from build123d import *

# Parameters (mm, degrees)
SKETCH1_W                       = 45
SKETCH1_H                       = 27
BOSS_EXTRUDE1_DEPTH             = 3
CUT_EXTRUDE1_REACH              = 28.41
SKETCH2_R                       = 1.75
SKETCH3_R                       = 3
CUT_EXTRUDE2_DEPTH              = 2
BOSS_EXTRUDE2_DEPTH             = 6
CUT_EXTRUDE6_REACH              = 37.992
CUT_EXTRUDE6_START              = -3
SKETCH12_R                      = 8.25
SKETCH15_R                      = 2.5
CUT_EXTRUDE7_DEPTH              = 6
SKETCH16_R                      = 1.15
SKETCH16_R_2                    = 12
BOSS_EXTRUDE5_DEPTH             = 2.5
CUT_EXTRUDE8_START              = -3.75
SKETCH17_W                      = 5.5
SKETCH17_H                      = 3
CUT_EXTRUDE8_DEPTH              = 82.37731478
BOSS_EXTRUDE6_START             = -9
SKETCH18_R                      = 1.75
BOSS_EXTRUDE6_DEPTH             = 5
SKETCH21_W                      = 11.5
SKETCH21_H                      = 33.5
SKETCH21_R                      = 1.75
BOSS_EXTRUDE7_DEPTH             = 5.5
CUT_EXTRUDE9_DEPTH              = 2
CHAMFER1_SIZE                   = 3
CHAMFER1_SIZE2                  = 5.196152423
FILLET1_R                       = 5
CUT_EXTRUDE10_REACH             = 74.347
SKETCH20_W                      = 4
SKETCH20_H                      = 8
CUT_EXTRUDE10_DIRECTION_2_DEPTH = 73.346820939
CHAMFER2_SIZE2                  = 3
CHAMFER2_SIZE                   = 20
CHAMFER3_SIZE2                  = 20
CHAMFER3_SIZE                   = 3


# Some blends are built 0.0001 mm under size
with BuildPart() as part:
    # Sketch1 → Boss-Extrude1 (new body)
    with BuildSketch(Plane(origin=(0, 0, 0), x_dir=(1, 0, 0), z_dir=(0, 1, 0))):
        Rectangle(SKETCH1_W, SKETCH1_H)
    extrude(amount=BOSS_EXTRUDE1_DEPTH)

    # Sketch2 → Cut-Extrude1 (cut, up to next)
    with BuildSketch(Plane(origin=(0, 3, 0), x_dir=(1, 0, 0), z_dir=(0, 1, 0)), mode=Mode.PRIVATE) as cut_extrude1_sk1:
        with Locations(Location((-10, 10, 0), (0, 0, 270))):
            Circle(SKETCH2_R)
    cut_extrude1_tool1 = extrude(cut_extrude1_sk1.sketch, amount=-CUT_EXTRUDE1_REACH, mode=Mode.PRIVATE) & part.part
    # Sketch2 → Cut-Extrude1 (cut, up to next)
    with BuildSketch(Plane(origin=(0, 3, 0), x_dir=(1, 0, 0), z_dir=(0, 1, 0)), mode=Mode.PRIVATE) as cut_extrude1_sk2:
        with Locations(Location((10, 10, 0), (0, 0, 270))):
            Circle(SKETCH2_R)
    cut_extrude1_tool2 = extrude(cut_extrude1_sk2.sketch, amount=-CUT_EXTRUDE1_REACH, mode=Mode.PRIVATE) & part.part
    # Sketch2 → Cut-Extrude1 (cut, up to next)
    with BuildSketch(Plane(origin=(0, 3, 0), x_dir=(1, 0, 0), z_dir=(0, 1, 0)), mode=Mode.PRIVATE) as cut_extrude1_sk3:
        with Locations(Location((10, -10, 0), (0, 0, 270))):
            Circle(SKETCH2_R)
    cut_extrude1_tool3 = extrude(cut_extrude1_sk3.sketch, amount=-CUT_EXTRUDE1_REACH, mode=Mode.PRIVATE) & part.part
    # Sketch2 → Cut-Extrude1 (cut, up to next)
    with BuildSketch(Plane(origin=(0, 3, 0), x_dir=(1, 0, 0), z_dir=(0, 1, 0)), mode=Mode.PRIVATE) as cut_extrude1_sk4:
        with Locations(Location((-10, -10, 0), (0, 0, 270))):
            Circle(SKETCH2_R)
    cut_extrude1_tool4 = extrude(cut_extrude1_sk4.sketch, amount=-CUT_EXTRUDE1_REACH, mode=Mode.PRIVATE) & part.part
    add(cut_extrude1_tool1.solids().sort_by_distance((-10, 3, -10))[0], mode=Mode.SUBTRACT)
    add(cut_extrude1_tool2.solids().sort_by_distance((10, 3, -10))[0], mode=Mode.SUBTRACT)
    add(cut_extrude1_tool3.solids().sort_by_distance((10, 3, 10))[0], mode=Mode.SUBTRACT)
    add(cut_extrude1_tool4.solids().sort_by_distance((-10, 3, 10))[0], mode=Mode.SUBTRACT)

    # Sketch3 → Cut-Extrude2 (cut)
    with BuildSketch(Plane(origin=(0, 3, 0), x_dir=(1, 0, 0), z_dir=(0, 1, 0))):
        with Locations(Location((-10, 10, 0), (0, 0, 270))):
            Circle(SKETCH3_R)
        with Locations(Location((10, 10, 0), (0, 0, 90))):
            Circle(SKETCH3_R)
        with Locations(Location((10, -10, 0), (0, 0, 270))):
            Circle(SKETCH3_R)
        with Locations(Location((-10, -10, 0), (0, 0, 90))):
            Circle(SKETCH3_R)
    extrude(amount=-CUT_EXTRUDE2_DEPTH, mode=Mode.SUBTRACT)

    # Sketch5 → Boss-Extrude2 (add, symmetric)
    with BuildSketch(Plane.XY):
        with BuildLine():
            Line((16.25, 3), (-16.25, 3))
            Line((-16.25, 3), (-16.25, 20))
            Line((-16.25, 20), (-6.25, 20))
            ThreePointArc((-6.25, 20), (0, 13.75), (6.25, 20))
            Line((6.25, 20), (16.25, 20))
            Line((16.25, 20), (16.25, 3))
        make_face()
    extrude(amount=BOSS_EXTRUDE2_DEPTH, both=True)

    # Sketch12 → Cut-Extrude6 (cut, up to next)
    with BuildSketch(Plane.XY.offset(CUT_EXTRUDE6_START), mode=Mode.PRIVATE) as cut_extrude6_sk1:
        with Locations((0, 20)):
            Circle(SKETCH12_R)
    cut_extrude6_tool1 = extrude(cut_extrude6_sk1.sketch, amount=-CUT_EXTRUDE6_REACH, mode=Mode.PRIVATE) & part.part
    cut_extrude6 = cut_extrude6_tool1.solids().sort_by_distance((0, 20, -3))[0]
    add(cut_extrude6, mode=Mode.SUBTRACT)

    # Mirror1: Cut-Extrude6 across plane
    add(cut_extrude6.mirror(Plane.XY), mode=Mode.SUBTRACT)

    # Sketch15 → Cut-Extrude7 (cut)
    with BuildSketch(Plane(origin=(0, 20, 0), x_dir=(1, 0, 0), z_dir=(0, 1, 0))):
        with Locations(Location((-11.25, 0, 0), (0, 0, 180))):
            Circle(SKETCH15_R)
        with Locations((11.25, 0)):
            Circle(SKETCH15_R)
    extrude(amount=-CUT_EXTRUDE7_DEPTH, mode=Mode.SUBTRACT)

    # Sketch16 → Boss-Extrude5 (add)
    with BuildSketch(Plane.ZY.offset(16.25)):
        Polygon((9, 3), (9, 0), (49, 0), (49, 40), (9, 40), (6, 40), (6, 20), (-6, 20), (-6, 3), align=None)
        with Locations((47, 2)):
            Circle(SKETCH16_R, mode=Mode.SUBTRACT)
        with Locations(Location((47, 38, 0), (0, 0, 180))):
            Circle(SKETCH16_R, mode=Mode.SUBTRACT)
        with Locations(Location((11, 38, 0), (0, 0, 180))):
            Circle(SKETCH16_R, mode=Mode.SUBTRACT)
        with Locations((29, 20)):
            Circle(SKETCH16_R_2, mode=Mode.SUBTRACT)
    boss_extrude5 = extrude(amount=BOSS_EXTRUDE5_DEPTH)

    # Sketch17 → Cut-Extrude8 (cut)
    with BuildSketch(Plane.ZY.offset(22.5).offset(CUT_EXTRUDE8_START)):
        with Locations((10.75, 1.5)):
            Rectangle(SKETCH17_W, SKETCH17_H)
    cut_extrude8 = extrude(amount=CUT_EXTRUDE8_DEPTH, mode=Mode.SUBTRACT)

    # Mirror2: Boss-Extrude5, Cut-Extrude8 across plane
    add(boss_extrude5.mirror(Plane(origin=(0, 0, 0), x_dir=(0, 0, 1), z_dir=(1, 0, 0))))
    add(cut_extrude8.mirror(Plane(origin=(0, 0, 0), x_dir=(0, 0, 1), z_dir=(1, 0, 0))), mode=Mode.SUBTRACT)

    # Sketch18 → Boss-Extrude6 (add)
    with BuildSketch(Plane(origin=(0, 0, -6), x_dir=(-1, 0, 0), z_dir=(0, 0, -1)).offset(BOSS_EXTRUDE6_START)):
        Polygon((-42.25, 33.5), (-30.75, 33.5), (-30.75, 6.5), (-18.75, 6.5), (-18.75, 0), (-42.25, 0), (-42.25, 6.5), align=None)
        with Locations((-36.5, 29)):
            Circle(SKETCH18_R, mode=Mode.SUBTRACT)
        with Locations(Location((-36.5, 11, 0), (0, 0, 180))):
            Circle(SKETCH18_R, mode=Mode.SUBTRACT)
    extrude(amount=-BOSS_EXTRUDE6_DEPTH)

    # Sketch21 → Boss-Extrude7 (add)
    with BuildSketch(Plane.XY.offset(8)):
        with Locations((36.5, 16.75)):
            Rectangle(SKETCH21_W, SKETCH21_H)
        with Locations(Location((36.5, 29, 0), (0, 0, 180))):
            Circle(SKETCH21_R, mode=Mode.SUBTRACT)
        with Locations((36.5, 11)):
            Circle(SKETCH21_R, mode=Mode.SUBTRACT)
    extrude(amount=BOSS_EXTRUDE7_DEPTH)

    # Sketch19 → Cut-Extrude9 (cut)
    with BuildSketch(Plane(origin=(0, 0, 3), x_dir=(-1, 0, 0), z_dir=(0, 0, -1))):
        Polygon((-39.848631561, 11), (-38.174315781, 8.1), (-34.825684219, 8.1), (-33.151368439, 11), (-34.825684219, 13.9), (-38.174315781, 13.9), align=None)
        Polygon((-39.848631561, 29), (-38.174315781, 26.1), (-34.825684219, 26.1), (-33.151368439, 29), (-34.825684219, 31.9), (-38.174315781, 31.9), align=None)
    extrude(amount=-CUT_EXTRUDE9_DEPTH, mode=Mode.SUBTRACT)

    # Chamfer1
    chamfer1_edges = [part.edges().sort_by_distance(p)[0] for p in [
        (42.25, 33.5, 8.25),
        (30.75, 33.5, 8.25),
    ]]
    chamfer1_side = [part.faces().sort_by_distance(p)[0] for p in [
        (36.5, 33.5, 8.25),
    ]]
    chamfer(chamfer1_edges, length=CHAMFER1_SIZE, length2=CHAMFER1_SIZE2, reference=chamfer1_side[0])

    # Fillet1
    # the kernel refuses this fillet: 5 mm, written as the material it takes off along each edge
    with BuildSketch(Plane(origin=(42.25, 0, -9.5), x_dir=(-1, 0, 0), z_dir=(0, 0, 1))) as fillet1_piece_1:
        with BuildLine():
            CenterArc((FILLET1_R, -FILLET1_R), FILLET1_R, 90, 90)
            Line((0, -FILLET1_R), (0, 0))
            Line((0, 0), (FILLET1_R, 0))
        make_face()
    extrude(amount=35.5, mode=Mode.SUBTRACT)
    with BuildSketch(Plane(origin=(42.25, 28.303847577, -0.349364905), x_dir=(-0.4999999999999988, 0.8660254037844394, 0), z_dir=(0, 0, 1))) as fillet1_piece_2:
        with BuildLine():
            CenterArc((FILLET1_R * 0.267949192431, FILLET1_R), FILLET1_R, 240, 30)
            Line((-FILLET1_R * 0.232050807569, FILLET1_R * 0.133974596216), (0, 0))
            Line((0, 0), (FILLET1_R * 0.267949192431, 0))
        make_face()
    extrude(amount=17.198729811, mode=Mode.SUBTRACT)
    with BuildSketch(Plane(origin=(30.75, 28.303847577, 16.849364905), x_dir=(0, -1, 0), z_dir=(0, 0, -1))) as fillet1_piece_3:
        with BuildLine():
            CenterArc((FILLET1_R * 0.267949192431, -FILLET1_R), FILLET1_R, 90, 30)
            Line((-FILLET1_R * 0.232050807569, -FILLET1_R * 0.133974596216), (0, 0))
            Line((0, 0), (FILLET1_R * 0.267949192431, 0))
        make_face()
    extrude(amount=17.198729811, mode=Mode.SUBTRACT)
    with BuildSketch(Plane(origin=(39.25, 33.5, -4.216878365), x_dir=(-1, 0, 0), z_dir=(0, 0, 1))) as fillet1_piece_4:
        with BuildLine():
            CenterArc((FILLET1_R * 0.57735026919, FILLET1_R), FILLET1_R, 210, 60)
            Line((-FILLET1_R * 0.288675134595, FILLET1_R * 0.5), (0, 0))
            Line((0, 0), (FILLET1_R * 0.57735026919, 0))
        make_face()
    extrude(amount=24.93375673, mode=Mode.SUBTRACT)
    with BuildSketch(Plane(origin=(33.75, 33.5, 20.716878365), x_dir=(-0.4999999999999974, -0.86602540378444, 0), z_dir=(0, 0, -1))) as fillet1_piece_5:
        with BuildLine():
            CenterArc((FILLET1_R * 0.57735026919, -FILLET1_R), FILLET1_R, 90, 60)
            Line((-FILLET1_R * 0.288675134595, -FILLET1_R * 0.5), (0, 0))
            Line((0, 0), (FILLET1_R * 0.57735026919, 0))
        make_face()
    extrude(amount=24.93375673, mode=Mode.SUBTRACT)

    # Sketch20 → Cut-Extrude10 (cut, up to next)
    with BuildSketch(Plane.XY.offset(6), mode=Mode.PRIVATE) as cut_extrude10_sk1:
        with Locations((-14.25, 7)):
            Rectangle(SKETCH20_W, SKETCH20_H)
    cut_extrude10_tool1 = extrude(cut_extrude10_sk1.sketch, amount=-CUT_EXTRUDE10_REACH, mode=Mode.PRIVATE) & part.part
    # Sketch20 → Cut-Extrude10 (cut, up to next)
    with BuildSketch(Plane.XY.offset(6), mode=Mode.PRIVATE) as cut_extrude10_sk2:
        with Locations((14.25, 7)):
            Rectangle(SKETCH20_W, SKETCH20_H)
    cut_extrude10_tool2 = extrude(cut_extrude10_sk2.sketch, amount=-CUT_EXTRUDE10_REACH, mode=Mode.PRIVATE) & part.part
    add(cut_extrude10_tool1.solids().sort_by_distance((-14.25, 7, 6))[0], mode=Mode.SUBTRACT)
    add(cut_extrude10_tool2.solids().sort_by_distance((14.25, 7, 6))[0], mode=Mode.SUBTRACT)

    # Sketch20 → Cut-Extrude10 direction 2 (cut)
    with BuildSketch(Plane.XY.offset(6)):
        with Locations((-14.25, 7)):
            Rectangle(SKETCH20_W, SKETCH20_H)
        with Locations((14.25, 7)):
            Rectangle(SKETCH20_W, SKETCH20_H)
    extrude(amount=CUT_EXTRUDE10_DIRECTION_2_DEPTH, mode=Mode.SUBTRACT)

    # Chamfer2
    chamfer2_edges = [part.edges().sort_by_distance(p)[0] for p in [
        (-17.5, 40, 6),
    ]]
    chamfer2_side = [part.faces().sort_by_distance(p)[0] for p in [
        (-17.5, 39.94, 6),
    ]]
    chamfer(chamfer2_edges, length=CHAMFER2_SIZE - 0.0001, length2=CHAMFER2_SIZE2 - 0.0001, reference=chamfer2_side[0])  # a hair under: the kernel refuses the full size

    # Chamfer3
    chamfer3_edges = [part.edges().sort_by_distance(p)[0] for p in [
        (17.5, 40, 6),
    ]]
    chamfer3_side = [part.faces().sort_by_distance(p)[0] for p in [
        (17.5, 40, 6.06),
    ]]
    chamfer(chamfer3_edges, length=CHAMFER3_SIZE - 0.0001, length2=CHAMFER3_SIZE2 - 0.0001, reference=chamfer3_side[0])  # a hair under: the kernel refuses the full size


solid = part.part
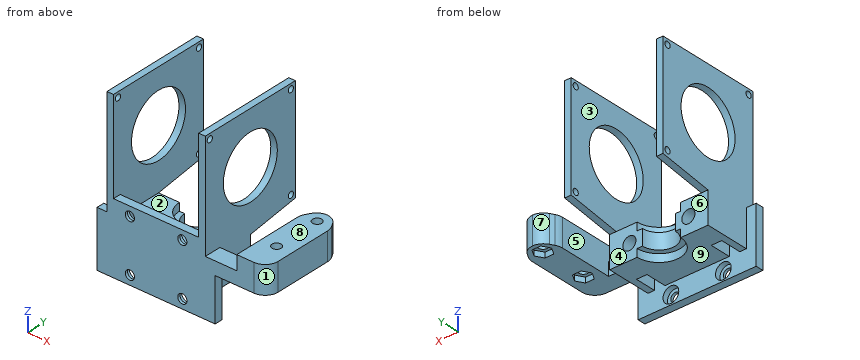
The model under review builds one solid part; all positions refer to its coordinate system, in mm. Face numbers are marked on the shaded views. A direction names the side the tool comes from. Coordinates: 2 decimals unless noted, no trailing zeros. Write each loop counter-clockwise with the first axis right and the second up, starting at its lowest first coordinate (ties: lowest second). Pieces come first, ordered by that corner, then holes. Notation, with made-up numbers: M -25.5,13.5 L 24.5,13.5 A21 ccw 24.5,49.5 Z; hole C 76.5,40.5 d7. An arc over 180 degrees is marked long. Put each result on its own line as item: value.
1) Add section B-B on z = 47. Give the boundary of the cut face in (x, y), then the cut area to 3 significant figures.
Computed:
outline: M -18.75,0 L -16.25,0 L -16.25,0.85 L -18.75,0.85 Z; M -18.75,3.15 L -16.25,3.15 L -16.25,36.85 L -18.75,36.85 Z; M -18.75,39.15 L -16.25,39.15 L -16.25,40 L -18.75,40 Z; M 16.25,0 L 18.75,0 L 18.75,0.85 L 16.25,0.85 Z; M 16.25,3.15 L 18.75,3.15 L 18.75,36.85 L 16.25,36.85 Z; M 16.25,39.15 L 18.75,39.15 L 18.75,40 L 16.25,40 Z
area: 177 mm2
2) Add section A-A on x = 10. Give the boundary of the cut face in (y, z), then the cut area to 3 significant figures.
Computed:
outline: M 0,-13.5 L 3,-13.5 L 3,-13 L 1,-13 L 1,-11.75 L 0,-11.75 Z; M 0,-8.25 L 1,-8.25 L 1,-7 L 3,-7 L 3,-6 L 20,-6 L 20,-2.17 L 14,-2.17 L 14,2.17 L 20,2.17 L 20,6 L 3,6 L 3,7 L 1,7 L 1,8.25 L 0,8.25 Z; M 0,11.75 L 1,11.75 L 1,13 L 3,13 L 3,13.5 L 0,13.5 Z
area: 228 mm2
3) For the marked faces 5, 6, 7, 8 and 9, list the 3-axis set-ups (+Z, -Z, +X, -X, +Y, -Y) from which the entire face can be reached by the end or side of a thin tool; tool diameter is ignored.
Computed:
face 5: +Z, +Y
face 6: -Z, -X, +Y
face 7: +Z, -Z, +Y
face 8: +Z, +X, +Y, -Y
face 9: -Z, +X, -X, +Y
4) Add section C-C on x = 0. Give the boundary of the cut face in (y, z), then the cut area to 3 significant figures.
Computed:
outline: M 0,-13.5 L 3,-13.5 L 3,-6 L 11.75,-6 L 11.75,-3 L 13.75,-3 L 13.75,3 L 11.75,3 L 11.75,6 L 3,6 L 3,13.5 L 0,13.5 Z
area: 198 mm2
5) Draft analysis for pull direction X (two halves, no side actions). For the marked faces 1, 2, 3 and 4, state which applies: released by +X, released by -X, zero draft, split by the parting line, or undercut.
Computed:
face 1: released by +X
face 2: undercut
face 3: undercut
face 4: zero draft
6) Wall thickness on probe 1 along X at (y, z) = (25, 13); probe 2 along X at (y, z) = (1.6, -10); probe 3 along Z at (x, y) = (10, 2): over which ranges is each line inside the solid? List them lowest first. Write a range as [from, to].
Computed:
probe 1: x = [-18.75, -16.25], [16.25, 18.75], [30.75, 42.25]
probe 2: x = [-22.5, -13], [-7, 7], [13, 22.5]
probe 3: z = [-13.5, -13], [-7, 7], [13, 13.5]
7) Add section D-D on y = 38. Give the boundary of the cut face in (x, z).
Computed:
outline: M -18.75,8.7 L -16.25,8.7 L -16.25,9.85 L -18.75,9.85 Z; M -18.75,12.15 L -16.25,12.15 L -16.25,45.85 L -18.75,45.85 Z; M -18.75,48.15 L -16.25,48.15 L -16.25,49 L -18.75,49 Z; M 16.25,8.7 L 18.75,8.7 L 18.75,9.85 L 16.25,9.85 Z; M 16.25,12.15 L 18.75,12.15 L 18.75,45.85 L 16.25,45.85 Z; M 16.25,48.15 L 18.75,48.15 L 18.75,49 L 16.25,49 Z
8) Clearance check with flat-ended pins moving along their axes: pin 1 Ø12 at (x, z) = (35.5, -1.5) entering from +Y; pin 2 Ø6 at (y, z) = (5.5, 34) entering from +X; pin 3 Ø4 at (x, y) = (6, 11.5) entering from -Z; pin 4 Ø1.8 at (y, z) = (2, 47) entering from -X. State where each tip first meets the part, or that it passes through.
Computed:
pin 1: stops at y = 33.5
pin 2: stops at x = 18.75
pin 3: stops at z = -6
pin 4: passes through
